Geometry check sheet. Reference: drawing and pictorial views, mm from the part's lowest x, y, z. A direction names the side the tool comes from. Give positions to 0.01 mm unless a question says otherwise; leave off trailing zeros. Write each loop counter-clockwise with the first axis right and the second up, starting at its lowest first coordinate (ties: lowest second). Pieces come first, ordered by that corner, then holes. Notation, with made-up numbers: (11, 76) - (24, 76) arc R29 cw to (24, 109) - close; hole circle Ø9 at (51, -17). An arc over 180 degrees is marked (long way). Write item = value, one per line. Start each with the question number.
(1) Draft check along Z on the marked faces 4 and 5. Enter one of: pulls with the +Z half, pulls with the -Z half, needs draft (parallel to the pull), parting line crosses it, or undercut.
(2) Access from +Z, -Z, +X, -X, +Y, -Y to the whole of each face (thin tool, end or side, straight path). Record for the marked faces 1, 2 and 3.
(3) Section check D-D, the plane z = 157.5. Enter the section's corners in (x, y), plus the area to 3 significant figures.
(4) Section check A-A, the plane z = 105. Enter the section's corners in (x, y).
(5) Depth check by flat-ended pin: pin 1 Ø8 at (x, z) = (102, 20) entering from +Y; pin 2 Ø21 at (x, z) = (103, 11) entering from -Y; pin 3 Ø21 at (x, z) = (162.85, 36.06) entering from -Y; pin 4 Ø1.5 at (x, y) = (59.5, 2.5) entering from -Z. Enter the tip coordinate at first touch or a pass-through.
(6) Thickness scan on L1, parallel to X at y = 6.75, z = 115.5; L2, parallel to X at y = 1.25, z = 34.5 (1 decimal); L3, parallel to Z at x = 157, y = 2 (1 decimal). Record the ranges inside material, lowest first.
(7) Section check C-C, the plane y = 1.5. Give the number of separate pieces and of enclosed holes in the cut face, plus the area to 3 significant figures.
(8) Section check B-B, the plane x = 105. Enter the section's corners in (y, z).
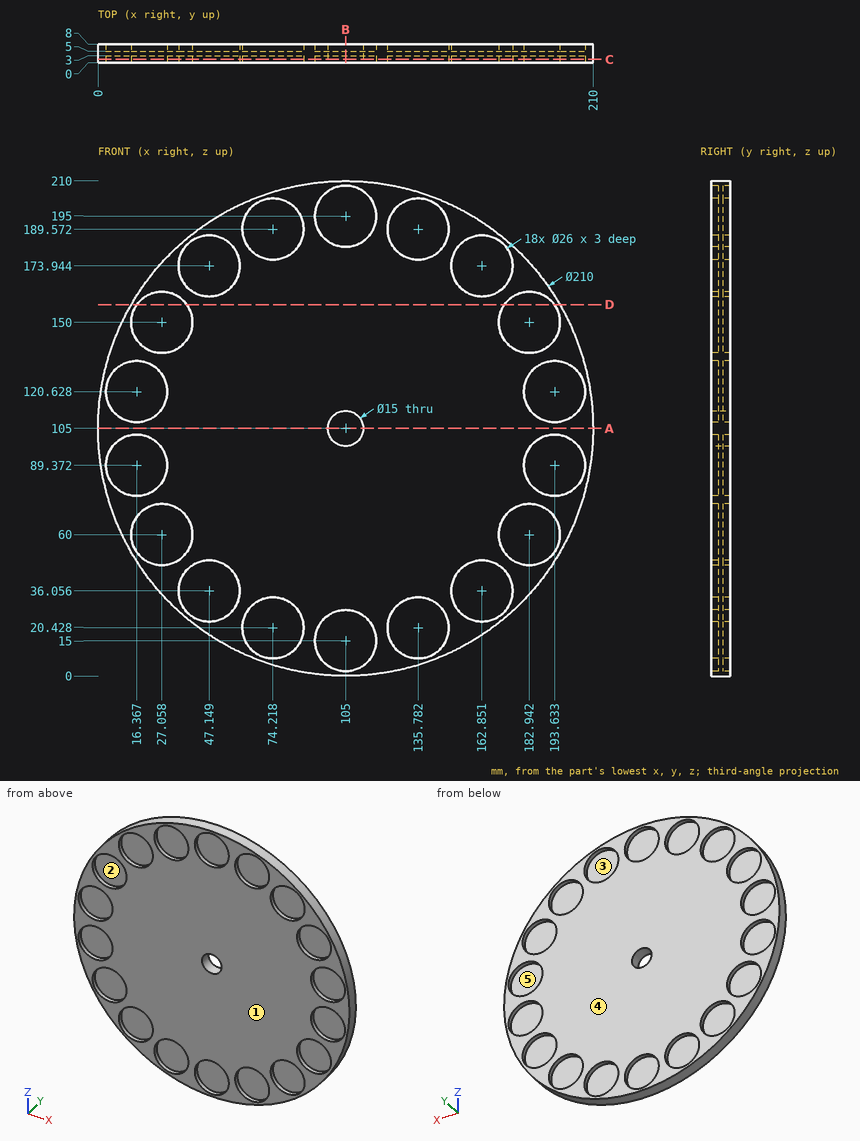
Model answer:
q1.face_4 = needs draft
q1.face_5 = undercut
q2.face_1 = +Z, -Z, +X, -X, -Y
q2.face_2 = -Y
q2.face_3 = +Y
q3.outline = (14.07, 0) - (16.44, 0) - (16.44, 3) - (37.68, 3) - (37.68, 0) - (172.32, 0) - (172.32, 3) - (193.56, 3) - (193.56, 0) - (195.93, 0) - (195.93, 8) - (193.56, 8) - (193.56, 5) - (172.32, 5) - (172.32, 8) - (37.68, 8) - (37.68, 5) - (16.44, 5) - (16.44, 8) - (14.07, 8) - close
q3.area = 1,200 mm²
q4.outline = (0, 0) - (97.5, 0) - (97.5, 8) - (0, 8) - close; (112.5, 0) - (210, 0) - (210, 8) - (112.5, 8) - close
q5.pin_1 = 5
q5.pin_2 = 0
q5.pin_3 = 3
q5.pin_4 = 10.01
q6.L1 = 0.53 to 4.42, 28.31 to 181.69, 205.58 to 209.47
q6.L2 = 27.2 to 34.2, 60.1 to 149.9, 175.8 to 182.8
q6.L3 = 13.8 to 24.4, 47.7 to 162.3, 185.6 to 196.2
q7.separate_pieces = 1
q7.enclosed_holes = 19
q7.area = 24,900 mm²
q8.outline = (0, 0) - (8, 0) - (8, 2) - (5, 2) - (5, 28) - (8, 28) - (8, 97.5) - (0, 97.5) - (0, 28) - (3, 28) - (3, 2) - (0, 2) - close; (0, 112.5) - (8, 112.5) - (8, 182) - (5, 182) - (5, 208) - (8, 208) - (8, 210) - (0, 210) - (0, 208) - (3, 208) - (3, 182) - (0, 182) - close
